Design review of the part built by this model. Coordinates are the model's own, in mm. Face numbers are marked on the shaded views. Round coordinates to 2 decimals unless told otherwise and drop trailing zeros. Order: outer loops, then holes, each group sorted by start corner. A loop starts at its lowest first (then second) coordinate and runs counter-clockwise, first axis right, second up. Notation, with made-up numbers: M 43,-15.75 L 61,-15.75 A34 ccw 61,16.25 Z; hole C 41,45.25 d6. An arc over 180 degrees is marked long. Use a Markdown table: item, result. Add a question column.
(1) The part is to be moulded in two halves that separate along X. For the marked faces 1, 2 and 3, say which applies: released by +X, released by -X, zero draft, split by the parting line, or undercut.
(2) To check wall thickness, follow probe 1 along X at (y, z) = (35.5, 15.5); probe 2 along X at (y, z) = (36.5, -15.5); probe 3 along Y at (x, z) = (11, 18). State the ranges of each line that lie inside material, in increasing order. Write a range as from..to.
(3) Take a section at B-B (y = 36.5). Write out the cut boundary in (x, z), then the cut area to 3 significant figures.
(4) Take a section at C-C (x = 0). Write out the cut boundary in (y, z), then the cut area to 3 significant figures.
(5) Take a section at A-A (z = 0). Write out the cut boundary in (x, y).
(6) For pin 1 (3 mm diameter, centred on x = 15.5, z = 15.5, fed in from +Y); pin 2 (3.5 mm diameter, centred on x = 15, z = 16, fed in from +Y); pin 3 (5 mm diameter, centred on y = 56, z = 4.5, fed in from +X), all flat-tipped, find the tip position at first contact; note any pin that passes through.
(7) Take a section at D-D (y = 26). Write out the cut boundary in (x, z), then the cut area to 3 significant figures.
```python
from build123d import *

# Parameters (mm, degrees)
SKETCH1_W           = 42
SKETCH1_H           = 42
BOSS_EXTRUDE1_DEPTH = 40
CHAMFER1_SIZE       = 5
SKETCH2_R           = 11
BOSS_EXTRUDE2_DEPTH = 2
SKETCH3_R           = 1.490042647
SKETCH3_R_2         = 1.56185503
SKETCH3_R_3         = 1.981129843
SKETCH3_R_4         = 1.582833873
CUT_EXTRUDE1_DEPTH  = 8
SKETCH4_R           = 2.5
BOSS_EXTRUDE3_DEPTH = 24


with BuildPart() as part:
    # Sketch1 → Boss-Extrude1 (new body)
    with BuildSketch(Plane(origin=(0, 0, 0), x_dir=(1, 0, 0), z_dir=(0, 1, 0))):
        Rectangle(SKETCH1_W, SKETCH1_H)
    extrude(amount=BOSS_EXTRUDE1_DEPTH)

    # Chamfer1
    chamfer1_edges = [part.edges().sort_by_distance(p)[0] for p in [
        (-21, 20, -21),
        (21, 20, -21),
        (21, 20, 21),
        (-21, 20, 21),
    ]]
    chamfer(chamfer1_edges, length=CHAMFER1_SIZE)

    # Sketch2 → Boss-Extrude2 (add)
    with BuildSketch(Plane(origin=(0, 40, 0), x_dir=(1, 0, 0), z_dir=(0, 1, 0))):
        Circle(SKETCH2_R)
    extrude(amount=BOSS_EXTRUDE2_DEPTH)

    # Sketch3 → Cut-Extrude1 (cut)
    with BuildSketch(Plane(origin=(0, 40, 0), x_dir=(1, 0, 0), z_dir=(0, 1, 0))):
        with Locations((15.5, 15.5)):
            Circle(SKETCH3_R)
        with Locations((15.5, -15.5)):
            Circle(SKETCH3_R_2)
        with Locations((-15.5, -15.5)):
            Circle(SKETCH3_R_3)
        with Locations((-15.5, 15.5)):
            Circle(SKETCH3_R_4)
    extrude(amount=-CUT_EXTRUDE1_DEPTH, mode=Mode.SUBTRACT)

    # Sketch4 → Boss-Extrude3 (add)
    with BuildSketch(Plane(origin=(0, 42, 0), x_dir=(1, 0, 0), z_dir=(0, 1, 0))):
        Circle(SKETCH4_R)
    extrude(amount=BOSS_EXTRUDE3_DEPTH)


solid = part.part
```
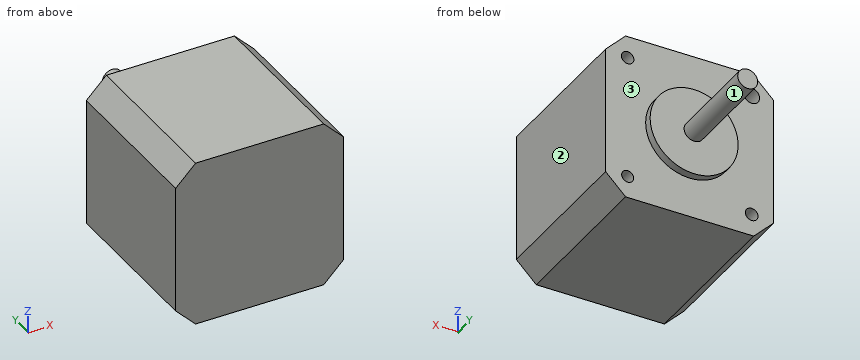
Verdict:
| question | item | result |
|---|---|---|
| 1 | face 1 | split by the parting line |
| 1 | face 2 | released by +X |
| 1 | face 3 | zero draft |
| 2 | probe 1 | x = -21..-17.48, -13.52..13.94, 17.06..21 |
| 2 | probe 2 | x = -21..-17.08, -13.92..14.01, 16.99..21 |
| 2 | probe 3 | y = 0..40 |
| 3 | outline | M -21,-16 L -16,-21 L 16,-21 L 21,-16 L 21,16 L 16,21 L -16,21 L -21,16 Z; hole C -15.5,15.5 d3.96; hole C -15.5,-15.5 d3.17; hole C 15.5,15.5 d3.12; hole C 15.5,-15.5 d2.98 |
| 3 | area | 1,680 mm^2 |
| 4 | outline | M 0,-21 L 40,-21 L 40,-11 L 42,-11 L 42,-2.5 L 66,-2.5 L 66,2.5 L 42,2.5 L 42,11 L 40,11 L 40,21 L 0,21 Z |
| 4 | area | 1,840 mm^2 |
| 5 | outline | M -21,0 L 21,0 L 21,40 L 11,40 L 11,42 L 2.5,42 L 2.5,66 L -2.5,66 L -2.5,42 L -11,42 L -11,40 L -21,40 Z |
| 6 | pin 1 | stops at y = 32 |
| 6 | pin 2 | stops at y = 40 |
| 6 | pin 3 | stops at x = 1.5 |
| 7 | outline | M -21,-16 L -16,-21 L 16,-21 L 21,-16 L 21,16 L 16,21 L -16,21 L -21,16 Z |
| 7 | area | 1,710 mm^2 |
